Source: three-view drawing plus pictorial views. Frame: mm from the lowest corner of the part. A direction names the side the tool comes from. Give positions to 0.01 mm unless a question says otherwise; leave off trailing zeros. Loops run counter-clockwise (first coordinate to the right, second up) from the corner with the lowest first, then second, coordinate; pieces in that order, holes last.
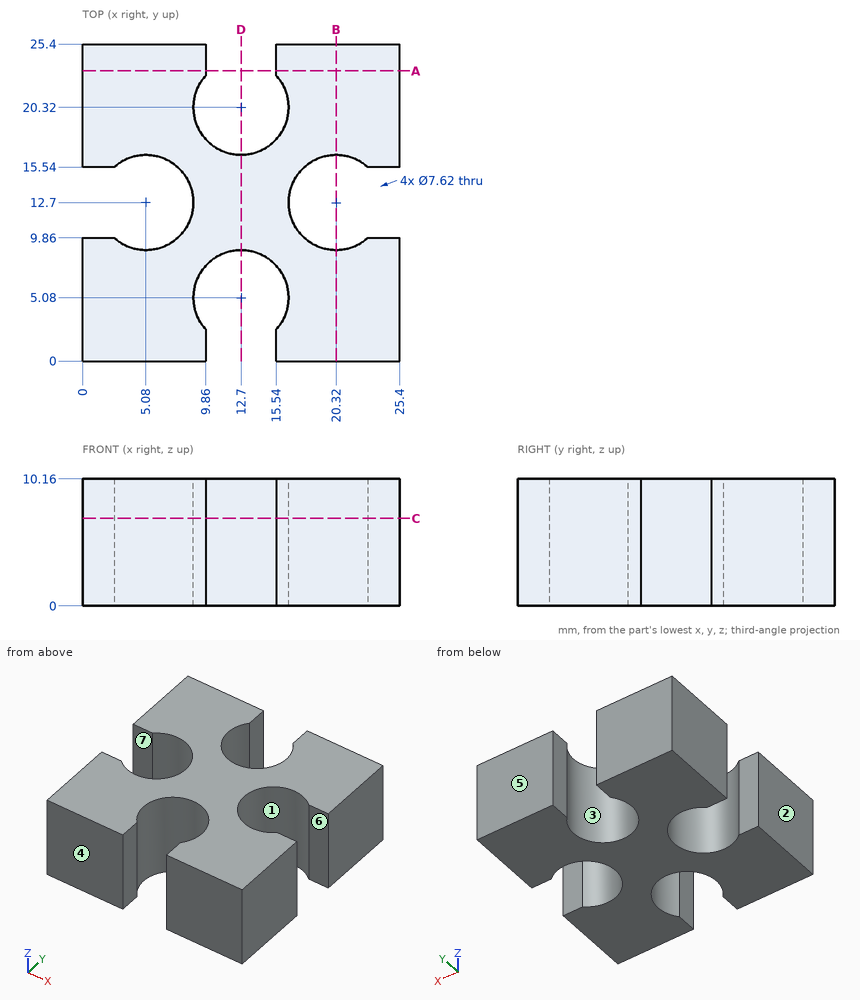
(1) Pin query (flat end, axial travel): pin 1 Ø6 at (x, y) = (5.08, 12.7) entering from -Z. Return the tip coordinate at first contact, or that it passes through.
Values follow:
pin 1: passes through
(2) Mould query, pull axis X, two halves, no side actions, for the marked faces 1, 2, 3 and 4. Classes: +X half, -X half, draft (parallel to the pull), parting line (faces both ways), or undercut.
Values follow:
face 1: undercut
face 2: -X half
face 3: undercut
face 4: draft
(3) Ray query, probe 1 along X at (y, z) = (20.32, 3.5); probe 2 along X at (y, z) = (16, 8.25) (1 decimal). Return the intervals inside material, ascending.
Values follow:
probe 1: x = 0 to 8.89, 16.51 to 25.4
probe 2: x = 0 to 3.2, 7 to 18.4, 22.2 to 25.4
(4) Cut plane C-C (z = 7). Return the cut outline in (x, y), and give its area (3 significant figures).
Values follow:
outline: (0, 0) - (9.86, 0) - (9.86, 2.54) arc R3.81 cw (long way) to (15.54, 2.54) - (15.54, 0) - (25.4, 0) - (25.4, 9.86) - (22.86, 9.86) arc R3.81 cw (long way) to (22.86, 15.54) - (25.4, 15.54) - (25.4, 25.4) - (15.54, 25.4) - (15.54, 22.86) arc R3.81 cw (long way) to (9.86, 22.86) - (9.86, 25.4) - (0, 25.4) - (0, 15.54) - (2.54, 15.54) arc R3.81 cw (long way) to (2.54, 9.86) - (0, 9.86) - close
area: 425 mm2
(5) Cut plane D-D (x = 12.7). Return the cut outline in (y, z).
Values follow:
outline: (8.89, 0) - (16.51, 0) - (16.51, 10.16) - (8.89, 10.16) - close
(6) Reachability of the marked faces 5, 6 and 7 from +Z, -Z, +X, -X, +Y, -Y: full face, straight path, thin tool, end or side. Return the list, or none.
Values follow:
face 5: +Z, -Z, +X, -X, +Y
face 6: +Z, -Z, +X
face 7: +Z, -Z, -X
(7) Cut plane A-A (y = 23.25). Return the cut outline in (x, z), and give its area (3 significant figures).
Values follow:
outline: (0, 0) - (9.86, 0) - (9.86, 10.16) - (0, 10.16) - close; (15.54, 0) - (25.4, 0) - (25.4, 10.16) - (15.54, 10.16) - close
area: 200 mm2
(8) Cut plane B-B (x = 20.32). Return the cut outline in (y, z), and give its area (3 significant figures).
Values follow:
outline: (0, 0) - (8.89, 0) - (8.89, 10.16) - (0, 10.16) - close; (16.51, 0) - (25.4, 0) - (25.4, 10.16) - (16.51, 10.16) - close
area: 181 mm2
